Autodesk Inventor part; units mm, degrees
ref_plane "YZ Plane" through (0, 0, 0) normal (1, 0, 0) x (0, 1, 0)
ref_plane "XZ Plane" through (0, 0, 0) normal (0, 1, 0) x (-1, 0, 0)
ref_plane "XY Plane" through (0, 0, 0) normal (0, 0, 1) x (1, 0, 0)
sketch "Sketch1" plane through (0, 0, 0) normal (0, 1, 0) x (-1, 0, 0)
  circle A0 centre (0, 0) radius 1.7
  line L0 (-3.5, 3.5) -> (3.5, 3.5)
  line L1 (3.5, 3.5) -> (3.5, -3.5)
  line L2 (3.5, -3.5) -> (-3.5, -3.5)
  line L3 (-3.5, -3.5) -> (-3.5, 3.5)
  line L4 (-3.5, 3.5) -> (3.5, -3.5) construction
  line L5 (3.5, 3.5) -> (-3.5, -3.5) construction
  dimension "d0" = 3.4
  dimension "d1" = 7
extrude "Extrusion1" add sketch "Sketch1" along normal blind 6
fillet "Fillet1" radius 2 4 edges at (3.5, 3, 3.5) (3.5, 3, -3.5) (-3.5, 3, -3.5) (-3.5, 3, 3.5)
properties part number "lcd_spacer"
The model under review builds one solid part; all positions refer to its coordinate system, in mm. Coordinates: 2 decimals unless noted, no trailing zeros. Loops run counter-clockwise (first coordinate to the right, second up) from the corner with the lowest first, then second, coordinate; pieces in that order, holes last. Notation, with made-up numbers: (-18.5, -4.5) -> (30.5, -4.5) arc R20 ccw to (30.5, 12.5) -> close; hole circle Ø9 at (51.25, 80). An arc over 180 degrees is marked (long way). Use a Markdown table: item, result. Add a question column.
1. Draft analysis for pull direction X (two halves, no side actions). For faces 1 (the face through (-3.5, 3, 0)), 2 (the face through (0.37, 2.96, 1.66)), 3 (the face through (2, 6, 1)), state which applies: pulls with the +X half, pulls with the -X half, needs draft (parallel to the pull), parting line crosses it, or undercut.
2. Add section C-C on y = 2.85. Write out the cut boundary in (x, z).
3. Add section B-B on x = 0. Write out the cut boundary in (y, z), plus the area to 3 significant figures.
4. Add section D-D on z = 2.75. Write out the cut boundary in (x, y).
5. To check wall thickness, follow line 1 (Z direction, x = 0, y = 1.6); line 2 (Z direction, x = -1, y = 2.75); line 3 (Z direction, x = -2.5, y = 2.55). State the ranges of each line that lie inside material, in increasing order.
6. Add section A-A on z = 0. Write out the cut boundary in (x, y), plus the area to 3 significant figures.
Returned:
| question | item | result |
|---|---|---|
| 1 | face 1 | pulls with the -X half |
| 1 | face 2 | undercut |
| 1 | face 3 | needs draft |
| 2 | outline | (-3.5, -1.5) arc R2 ccw to (-1.5, -3.5) -> (1.5, -3.5) arc R2 ccw to (3.5, -1.5) -> (3.5, 1.5) arc R2 ccw to (1.5, 3.5) -> (-1.5, 3.5) arc R2 ccw to (-3.5, 1.5) -> close; hole circle Ø3.4 at (0, 0) |
| 3 | outline | (0, -3.5) -> (6, -3.5) -> (6, -1.7) -> (0, -1.7) -> close; (0, 1.7) -> (6, 1.7) -> (6, 3.5) -> (0, 3.5) -> close |
| 3 | area | 21.6 mm² |
| 4 | outline | (-3.06, 0) -> (3.06, 0) -> (3.06, 6) -> (-3.06, 6) -> close |
| 5 | line 1 | z = -3.5 to -1.7, 1.7 to 3.5 |
| 5 | line 2 | z = -3.5 to -1.37, 1.37 to 3.5 |
| 5 | line 3 | z = -3.23 to 3.23 |
| 6 | outline | (-3.5, 0) -> (-1.7, 0) -> (-1.7, 6) -> (-3.5, 6) -> close; (1.7, 0) -> (3.5, 0) -> (3.5, 6) -> (1.7, 6) -> close |
| 6 | area | 21.6 mm² |
